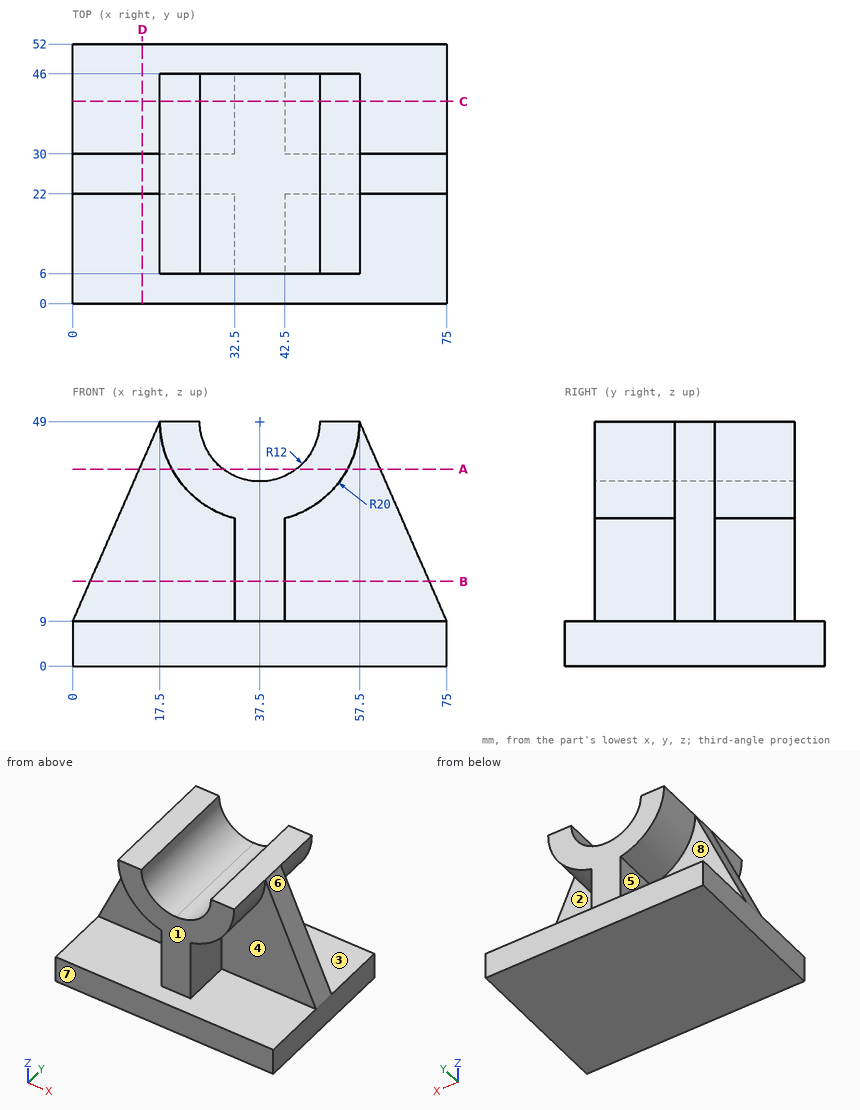
Print and shaded views of the part. All mm, measured from the part's lowest x, y and z. A direction names the side the tool comes from. Give positions to 0.01 mm unless a question says otherwise; leave off trailing zeros. Order: outer loops, then holes, each group sorted by start corner. A loop starts at its lowest first (then second) coordinate and runs counter-clockwise, first axis right, second up. Notation, with made-up numbers: (87, 45) - (97, 45) arc R26 ccw to (97, 67) - close; hole circle Ø2 at (73, 56). An arc over 180 degrees is marked (long way). Use a Markdown table: item, result.
1) Flat gauge pins, fed straight in: P1, Ø16, axis at x = 52.5, z = 22.5, coming from the +Y side; P2, Ø1, axis at x = 55, y = 33.5, coming from the -Z side; P3, Ø5, axis at y = 39, z = 18, coming from the +X side; P4, Ø10, axis at y = 11.5, z = 20, coming from the -X side. Where does each tip first touch, or does it go through?
Checked values:
| item | result |
|---|---|
| P1 | y = 30 |
| P2 | z = 0 |
| P3 | x = 42.5 |
| P4 | x = 32.5 |
2) Saw through at D-D on x = 14. List the corners of the cut face in (y, z), plus the area to 3 significant figures.
Checked values:
| item | result |
|---|---|
| outline | (0, 0) - (52, 0) - (52, 9) - (30, 9) - (30, 41) - (22, 41) - (22, 9) - (0, 9) - close |
| area | 724 mm² |
3) Two-plate mould, pull along Z, no slides. Class the marked faces 6, 7 and 8: +Z half, -Z half, draft (parallel to the pull), parting line (faces both ways), or undercut.
Checked values:
| item | result |
|---|---|
| face 6 | +Z half |
| face 7 | draft |
| face 8 | undercut |
4) 3-axis set-ups, long thin cutter, end or side, ignore diameter. For the marked faces 1, 2, 3, 4 and 5: which of +Z, -Z, +X, -X, +Y, -Y reach the whole face in a straight line?
Checked values:
| item | result |
|---|---|
| face 1 | +Z, +X, -X, -Y |
| face 2 | +X, +Y |
| face 3 | +Y |
| face 4 | +X, -Y |
| face 5 | -X, +Y |
5) Saw through at C-C on y = 40.5. List the corners of the cut face in (x, z).
Checked values:
| item | result |
|---|---|
| outline | (0, 0) - (75, 0) - (75, 9) - (42.5, 9) - (42.5, 29.64) arc R20 ccw to (57.5, 49) - (49.5, 49) arc R12 cw to (37.5, 37) arc R12 cw to (25.5, 49) - (17.5, 49) arc R20 ccw to (32.5, 29.64) - (32.5, 9) - (0, 9) - close |
6) Probe L1, parallel to Y at x = 54, z = 11; L2, parallel to X at y = 21, z = 15.5; L3, parallel to Z at x = 72, y = 41. List the from-to ranges inside material, lowest first. Write a range as from..to.
Checked values:
| item | result |
|---|---|
| L1 | 22..30 |
| L2 | 32.5..42.5 |
| L3 | 0..9 |
7) Saw through at A-A on z = 39.5. List the corners of the cut face in (x, y), plus the area to 3 significant figures.
Checked values:
| item | result |
|---|---|
| outline | (13.34, 22) - (19.9, 22) - (19.9, 6) - (30.17, 6) - (30.17, 46) - (19.9, 46) - (19.9, 30) - (13.34, 30) - close; (44.83, 6) - (55.1, 6) - (55.1, 22) - (61.66, 22) - (61.66, 30) - (55.1, 30) - (55.1, 46) - (44.83, 46) - close |
| area | 926 mm² |
8) Saw through at B-B on z = 17. List the corners of the cut face in (x, y).
Checked values:
| item | result |
|---|---|
| outline | (3.5, 22) - (32.5, 22) - (32.5, 6) - (42.5, 6) - (42.5, 22) - (71.5, 22) - (71.5, 30) - (42.5, 30) - (42.5, 46) - (32.5, 46) - (32.5, 30) - (3.5, 30) - close |
